Build history of the part. All positions in model axes, mm. A direction names the side the tool comes from. Give positions to 0.01 mm unless a question says otherwise; leave off trailing zeros. Loops run counter-clockwise (first coordinate to the right, second up) from the corner with the lowest first, then second, coordinate; pieces in that order, holes last. Notation, with made-up numbers: M 20,-31 L 72,-31 A27 cw 72,-10 Z; hole C 71.5,73.25 d9. An arc over 180 degrees is marked long. Answer as a JSON object with one key per item and string values. Group by question number.
1. 3-axis set-ups, long thin cutter, end or side, ignore diameter. For faces 1 (the face through (6, 83.185, 64)), 2 (the face through (0, 56, 21)): which of +Z, -Z, +X, -X, +Y, -Y reach the whole face in a straight line?
2. Slice it at A-A (z = 27). List the corners of the cut face in (x, y), then the cut area to 3 significant figures.
3. Drop flat-ended pins along their axis: pin 1 Ø2 at (x, y) = (6, 25) entering from +Z; pin 2 Ø10 at (y, z) = (39.5, 27.5) entering from +X; pin 3 Ø5 at (x, y) = (11, 11) entering from +Z; pin 4 Ø4 at (x, z) = (9, 48.5) entering from -Y. Give the stop position or say it passes through.
4. Mould opens along Y. For faces 3 (the face through (6, 47.942, 48)), 4 (the face through (12.7, 56, 21)), 5 (the face through (6.26, 88.21, 74.77)) say: released by +Y, released by -Y, zero draft, split by the parting line, or undercut.
5. Drill centre lines: line 1 along Y through (x, z) = (3.75, 63) (1 decimal); line 2 along Y through (x, z) = (7.5, 43.5); line 3 along Y through (x, z) = (5, 36.5). Where is each one in solid material? Low to high. Write a range as [from, to].
6. Slice it at D-D (y = 56.5). List the corners of the cut face in (x, z).
7. Slice it at C-C (z = 36.5). List the corners of the cut face in (x, y), then the cut area to 3 significant figures.
from build123d import *

# Parameters (mm, degrees)
F1_DEPTH = 12.7


with BuildPart() as f1:
    # F0 (on Right) → F1 (new body)
    with BuildSketch(Plane.YZ):
        with BuildLine():
            Line((0, 38.1), (0, 0))
            Line((0, 0), (93.0275, 0))
            Line((93.0275, 0), (93.0275, 69.85))
            ThreePointArc((93.0275, 69.85), (88.10625, 74.77125), (83.185, 69.85))
            Line((83.185, 69.85), (83.185, 57.15))
            ThreePointArc((83.185, 57.15), (70.485, 44.45), (57.785, 57.15))
            ThreePointArc((57.785, 57.15), (52.86375, 62.07125), (47.9425, 57.15))
            Line((47.9425, 57.15), (47.9425, 38.1))
            ThreePointArc((47.9425, 38.1), (28.8925, 19.05), (9.8425, 38.1))
            ThreePointArc((9.8425, 38.1), (4.92125, 43.02125), (0, 38.1))
        make_face()
    extrude(amount=F1_DEPTH)


solid = f1.part
Established:
{
 "1": {"face 1": "+Z, +X, -X", "face 2": "+Z, -Z, -X, +Y, -Y"},
 "2": {"outline": "M 0,0 L 12.7,0 L 12.7,13.41 L 0,13.41 Z; M 0,44.37 L 12.7,44.37 L 12.7,93.03 L 0,93.03 Z", "area": "788 mm^2"},
 "3": {"pin 1": "stops at z = 19.69", "pin 2": "stops at x = 12.7", "pin 3": "stops at z = 41.48", "pin 4": "stops at y = 47.94"},
 "4": {"face 3": "undercut", "face 4": "zero draft", "face 5": "split by the parting line"},
 "5": {"line 1": "y = [83.2, 93]", "line 2": "y = [47.94, 93.03]", "line 3": "y = [0, 9.91], [47.88, 93.03]"},
 "6": {"outline": "M 0,0 L 12.7,0 L 12.7,60.47 L 0,60.47 Z"},
 "7": {"outline": "M 0,0 L 12.7,0 L 12.7,9.91 L 0,9.91 Z; M 0,47.88 L 12.7,47.88 L 12.7,93.03 L 0,93.03 Z", "area": "699 mm^2"}
}
